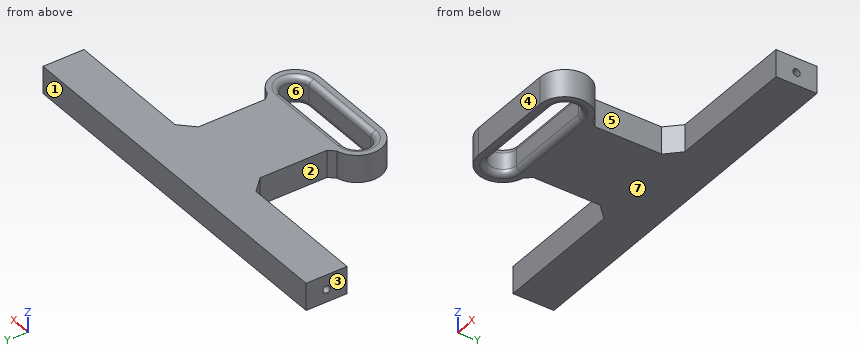
from build123d import *

# Parameters (mm, degrees)
PAD_DEPTH       = 10
SKETCH001_R     = 1.325
HOLE_DEPTH      = 15.20386
HOLE_TIPS_R     = 1.325
SKETCH002_R     = 1.325
HOLE001_DEPTH   = 15.20386
HOLE001_TIPS_R  = 1.325
FILLET_R        = 2
CHAMFER_SIZE    = 2
CHAMFER001_SIZE = 5


with BuildPart() as part:
    # Sketch → Pad (new body)
    with BuildSketch(Plane.XY):
        with BuildLine():
            Line((0, 15), (136.4, 15))
            Line((136.4, 15), (136.4, 0))
            Line((136.4, 0), (84.2, 0))
            Line((84.2, 0), (84.2, -31.5))
            ThreePointArc((84.2, -49.5), (93.2, -40.5), (84.2, -31.5))
            Line((52.2, -49.5), (84.2, -49.5))
            ThreePointArc((52.2, -31.5), (43.2, -40.5), (52.2, -49.5))
            Line((52.2, 0), (52.2, -31.5))
            Line((52.2, 0), (0, 0))
            Line((0, 0), (0, 15))
        make_face()
        with BuildLine():
            ThreePointArc((52.2, -35.5), (47.2, -40.5), (52.2, -45.5))
            Line((52.2, -45.5), (84.2, -45.5))
            ThreePointArc((84.2, -45.5), (89.2, -40.5), (84.2, -35.5))
            Line((52.2, -35.5), (84.2, -35.5))
        make_face(mode=Mode.SUBTRACT)
    extrude(amount=PAD_DEPTH)

    # Sketch001 (on Face2 of Pad) → Hole (cut)
    with BuildSketch(Plane(origin=(0, 0, 0), x_dir=(0, -1, 0), z_dir=(-1, 0, 0))):
        with Locations((-7.5, 4.65)):
            Circle(SKETCH001_R)
    extrude(amount=-HOLE_DEPTH, mode=Mode.SUBTRACT)

    # Hole tips → Hole tip 1 section 0
    with BuildSketch(Plane(origin=(15.20386, 0, 0), x_dir=(0, -1, 0), z_dir=(-1, 0, 0)), mode=Mode.PRIVATE) as hole_tip_1_s0:
        with Locations((-7.5, 4.65)):
            Circle(HOLE_TIPS_R)
    loft([hole_tip_1_s0.sketch, Vertex(16, 7.5, 4.65)], mode=Mode.SUBTRACT)

    # Sketch002 (on Face4 of Pad) → Hole001 (cut)
    with BuildSketch(Plane.YZ.offset(136.4)):
        with Locations((7.5, 4.65)):
            Circle(SKETCH002_R)
    extrude(amount=-HOLE001_DEPTH, mode=Mode.SUBTRACT)

    # Hole001 tips → Hole001 tip 1 section 0
    with BuildSketch(Plane.YZ.offset(121.19614), mode=Mode.PRIVATE) as hole001_tip_1_s0:
        with Locations((7.5, 4.65)):
            Circle(HOLE001_TIPS_R)
    loft([hole001_tip_1_s0.sketch, Vertex(120.4, 7.5, 4.65)], mode=Mode.SUBTRACT)

    # Fillet
    fillet_edges = [part.edges().sort_by_distance(p)[0] for p in [
        (68.2, -35.5, 10),
        (89.2, -40.5, 10),
        (47.2, -40.5, 10),
        (68.2, -45.5, 10),
        (68.2, -35.5, 0),
        (89.2, -40.5, 0),
        (68.2, -45.5, 0),
        (47.2, -40.5, 0),
    ]]
    fillet(fillet_edges, radius=FILLET_R)

    # Chamfer
    chamfer_edges = [part.edges().sort_by_distance(p)[0] for p in [
        (52.2, -31.5, 5),
        (84.2, -31.5, 5),
    ]]
    chamfer(chamfer_edges, length=CHAMFER_SIZE)

    # Chamfer001
    chamfer001_edges = [part.edges().sort_by_distance(p)[0] for p in [
        (52.2, 0, 5),
        (84.2, 0, 5),
    ]]
    chamfer(chamfer001_edges, length=CHAMFER001_SIZE)


solid = part.part
Input: part model. Units: mm. Frame: model coordinates. Face numbers are marked on the shaded views. A direction names the side the tool comes from. Give positions to 0.01 mm unless a question says otherwise; leave off trailing zeros. Write each loop counter-clockwise with the first axis right and the second up, starting at its lowest first coordinate (ties: lowest second). Pieces come first, ordered by that corner, then holes.
Q1. First-contact query: P1, Ø2, axis at y = 7.5, z = 4.65, coming from the -X side; P2, Ø5, axis at x = 98, z = 7.5, coming from the -Y side; P3, Ø4, axis at y = -34.5, z = 4.5, coming from the +X side. Flat tips, straight axial feed; report the tip coordinate or a pass-through.
Q2. Section C-C, the plane x = 37. Output: boundary loops of the cut face in (y, z).
Q3. Material intervals for probe 1 along Z at (x, y) = (8, 7.5) (3 decimals); probe 2 along Y at (x, z) = (88, 8.5); probe 3 along Y at (x, z) = (87.5, 9.5), sorted ascending.
Q4. Section A-A, the plane x = 57.5. Output: boundary loops of the cut face in (y, z).
Q5. Section D-D, the plane y = -2. Output: boundary loops of the cut face in (x, z), plus the area to 3 significant figures.
Q6. Set-up query: the marked faces 5, 6 and 7. Return all of +Z, -Z, +X, -X, +Y, -Y with unobstructed straight access to the full face (end or side cutting, diameter ignored); none if empty.
Q7. Pull-direction query (Y, two-part tool) for the marked faces 1, 2, 3 and 4; classes: pulls with the +Y half, pulls with the -Y half, needs draft (parallel to the pull), parting line crosses it, or undercut.
Q8. Section B-B, the plane y = -40.5. Output: boundary loops of the cut face in (x, z), plus the area to 3 significant figures.
Filled in:
1. P1: stops at x = 15.4
1. P2: stops at y = 0
1. P3: stops at x = 92.26
2. outline: (0, 0) - (15, 0) - (15, 10) - (0, 10) - close
3. probe 1: z = 0 to 3.325, 5.975 to 10
3. probe 2: y = -48.66 to -43.85, -37.15 to -32.34, -1.2 to 15
3. probe 3: y = -48.87 to -45.12, -35.88 to -32.13, -1.7 to 15
4. outline: (-49.5, 0) - (-47.5, 0) arc R2 ccw to (-45.5, 2) - (-45.5, 8) arc R2 ccw to (-47.5, 10) - (-49.5, 10) - close; (-35.5, 2) arc R2 ccw to (-33.5, 0) - (15, 0) - (15, 10) - (-33.5, 10) arc R2 ccw to (-35.5, 8) - close
5. outline: (49.2, 0) - (87.2, 0) - (87.2, 10) - (49.2, 10) - close
5. area: 380 mm2
6. face 5: +Z, -Z, +X
6. face 6: +Z, -Z
6. face 7: -Z, +X, -X, +Y, -Y
7. face 1: pulls with the +Y half
7. face 2: undercut
7. face 3: needs draft
7. face 4: pulls with the -Y half
8. outline: (43.2, 0) - (45.2, 0) arc R2 ccw to (47.2, 2) - (47.2, 8) arc R2 ccw to (45.2, 10) - (43.2, 10) - close; (89.2, 2) arc R2 ccw to (91.2, 0) - (93.2, 0) - (93.2, 10) - (91.2, 10) arc R2 ccw to (89.2, 8) - close
8. area: 76.6 mm2
